Verification items for the finished model (mm, model axes). A direction names the side the tool comes from. Give positions to 0.01 mm unless a question says otherwise; leave off trailing zeros. Order: outer loops, then holes, each group sorted by start corner. A loop starts at its lowest first (then second) coordinate and runs counter-clockwise, first axis right, second up.
(1) Gauge pin test, flat ends, axial feed: pin 1 (1.5 mm diameter, centred on x = -4, z = 6, fed in from +Y); pin 2 (0.5 mm diameter, centred on y = 4.5, z = 4, fed in from -X); pin 3 (1 mm diameter, centred on y = 2, z = 3.5, fed in from +X); pin 4 (2 mm diameter, centred on x = 0, z = 5, fed in from -Y). Record the tip position at first contact, or that the pin passes through.
(2) Mould release check, pull along Z, two halves, no side actions. Record for faces 4 (the face through (-3.946, 1.913, 0.06)), 5 (the face through (-4.02, 1.94, 4.93)), 6 (the face through (0.27, 2.47, 6.22)), 7 (the face through (-3.946, 1.913, 9.94)): pulls with the +Z half, pulls with the -Z half, needs draft (parallel to the pull), parting line crosses it, or undercut.
(3) Sectioned sample at A-A on y = 4.4. Record the cut outline in (x, z), plus the area to 3 significant figures.
(4) Scan lines: L1, parallel to Z at x = 0, y = 3.4; L2, parallel to X at y = 2.7, z = 5; L3, parallel to Z at x = -1, y = 2.85. Record each from-to range of solid material in increasing order.
(5) Sectioned sample at C-C on z = 5. Record the cut outline in (x, y), plus the area to 3 significant figures.
(6) Sectioned sample at B-B on x = 0. Record the cut outline in (y, z).
(7) Sectioned sample at D-D on z = 8.5. Record the cut outline in (x, y), plus the area to 3 significant figures.
(8) Access from +Z, -Z, +X, -X, +Y, -Y to the whole of each face (thin tool, end or side, straight path). Record for faces 1 (the face through (-4, 4, 5)), 2 (the face through (4, 4, 5)), 3 (the face through (0, 3, 10)).
```python
from build123d import *

# Parameters (mm, degrees)
NUTEXTRUSION_DEPTH    = 10
M3X0_5_TAPPED_HOLE1_D = 2.5
COSMETIC_FILLETS_R    = 0.2


with BuildPart() as part:
    # MainSketch → NutExtrusion (new body)
    with BuildSketch(Plane.XY):
        Polygon((-3.1, 0), (3.1, 0), (5, 4), (3.1, 4), (3.1, 5), (-3.1, 5), (-3.1, 4), (-5, 4), align=None)
    extrude(amount=NUTEXTRUSION_DEPTH)

    # M3x0.5 Tapped Hole1 (through all)
    with Locations(Plane(origin=(0, 5, 0), x_dir=(1, 0, 0), z_dir=(0, 1, 0))):
        with Locations((0, -5)):
            Hole(M3X0_5_TAPPED_HOLE1_D / 2)

    # Cosmetic Fillets
    cosmetic_fillets_edges = [part.edges().sort_by_distance(p)[0] for p in [
        (4.05, 4, 0),
        (3.1, 4, 5),
        (3.1, 4.5, 0),
        (3.1, 5, 5),
        (0, 5, 0),
        (-3.1, 5, 5),
        (1.25, 5, 5),
        (1.25, 0, 5),
        (-3.1, 4.5, 0),
        (-3.1, 4, 5),
        (-4.05, 4, 0),
        (-5, 4, 5),
        (-4.05, 2, 0),
        (-3.1, 0, 5),
        (0, 0, 0),
        (0, 0, 10),
        (4.05, 2, 10),
        (4.05, 4, 10),
        (3.1, 4.5, 10),
        (0, 5, 10),
        (-3.1, 4.5, 10),
        (-4.05, 4, 10),
        (-4.05, 2, 10),
        (3.1, 0, 5),
        (4.05, 2, 0),
        (5, 4, 5),
    ]]
    fillet(cosmetic_fillets_edges, radius=COSMETIC_FILLETS_R)


solid = part.part
```
Ans:
1. pin 1: stops at y = 4.01
1. pin 2: stops at x = -3.1
1. pin 3: stops at x = 4.29
1. pin 4: passes through
2. face 4: pulls with the -Z half
2. face 5: needs draft
2. face 6: undercut
2. face 7: pulls with the +Z half
3. outline: (-3.1, 0.2) arc R0.2 ccw to (-2.9, 0) - (2.9, 0) arc R0.2 ccw to (3.1, 0.2) - (3.1, 9.8) arc R0.2 ccw to (2.9, 10) - (-2.9, 10) arc R0.2 ccw to (-3.1, 9.8) - close; hole circle Ø2.5 at (0, 5)
3. area: 57.1 mm2
4. L1: z = 0 to 3.75, 6.25 to 10
4. L2: x = -4.38 to -1.25, 1.25 to 4.38
4. L3: z = 0 to 4.25, 5.75 to 10
5. outline: (-4.86, 3.71) - (-3.15, 0.11) arc R0.2 ccw to (-2.97, 0) - (-1.45, 0) arc R0.2 ccw to (-1.25, 0.2) - (-1.25, 4.8) arc R0.2 ccw to (-1.45, 5) - (-2.9, 5) arc R0.2 ccw to (-3.1, 4.8) - (-3.1, 4.2) arc R0.2 cw to (-3.3, 4) - (-4.68, 4) arc R0.2 ccw to start; (1.25, 0.2) arc R0.2 ccw to (1.45, 0) - (2.97, 0) arc R0.2 ccw to (3.15, 0.11) - (4.86, 3.71) arc R0.2 ccw to (4.68, 4) - (3.3, 4) arc R0.2 cw to (3.1, 4.2) - (3.1, 4.8) arc R0.2 ccw to (2.9, 5) - (1.45, 5) arc R0.2 ccw to (1.25, 4.8) - close
5. area: 26.0 mm2
6. outline: (0, 0.2) arc R0.2 ccw to (0.2, 0) - (4.8, 0) arc R0.2 ccw to (5, 0.2) - (5, 3.55) arc R0.2 ccw to (4.8, 3.75) - (0.2, 3.75) arc R0.2 ccw to (0, 3.55) - close; (0, 6.45) arc R0.2 ccw to (0.2, 6.25) - (4.8, 6.25) arc R0.2 ccw to (5, 6.45) - (5, 9.8) arc R0.2 ccw to (4.8, 10) - (0.2, 10) arc R0.2 ccw to (0, 9.8) - close
7. outline: (-4.86, 3.71) - (-3.15, 0.11) arc R0.2 ccw to (-2.97, 0) - (2.97, 0) arc R0.2 ccw to (3.15, 0.11) - (4.86, 3.71) arc R0.2 ccw to (4.68, 4) - (3.3, 4) arc R0.2 cw to (3.1, 4.2) - (3.1, 4.8) arc R0.2 ccw to (2.9, 5) - (-2.9, 5) arc R0.2 ccw to (-3.1, 4.8) - (-3.1, 4.2) arc R0.2 cw to (-3.3, 4) - (-4.68, 4) arc R0.2 ccw to start
7. area: 38.5 mm2
8. face 1: +Z, -Z, -X, +Y
8. face 2: +Z, -Z, +X, +Y
8. face 3: +Z, +X, -X, +Y, -Y
